from build123d import *

# Parameters (mm, degrees)
SKETCH1_R           = 3.425
HUB_DEPTH           = 2.4
SKETCH2_R           = 0.4
BOSS_EXTRUDE2_DEPTH = 1.8
SKETCH3_R           = 2.15
CUT_EXTRUDE1_DEPTH  = 0.8
SKETCH4_R           = 1.2
CUT_EXTRUDE2_DEPTH  = 17.520612
CUT_EXTRUDE3_START  = -3
CUT_EXTRUDE3_DEPTH  = 3
CIRPATTERN1_COUNT   = 20
CUT_EXTRUDE4_START  = -3
SKETCH6_R           = 2.15
CUT_EXTRUDE4_DEPTH  = 3


with BuildPart() as part:
    # Sketch1 → HUB (new body)
    with BuildSketch(Plane(origin=(0, 0, 0), x_dir=(1, 0, 0), z_dir=(0, 1, 0))):
        with Locations(Location((0, 0, 0), (0, 0, 270))):
            Circle(SKETCH1_R)
    extrude(amount=HUB_DEPTH)

    # Sketch2 → Boss-Extrude2 (add)
    with BuildSketch(Plane(origin=(0, 2.4, 0), x_dir=(1, 0, 0), z_dir=(0, 1, 0))):
        with BuildLine():
            Line((-2.875, 1.861451), (-1.85, 14))
            add(Edge.make_bspline(
                [(-1.85, 14), (-1.761904, 15.043277), (-0.882336, 15.809649), (0.882387, 15.802355), (1.755744, 15.11622), (1.85, 14)],
                knots=[0, 0, 0, 0, 0.45, 0.55, 1, 1, 1, 1], degree=3))
            Line((1.85, 14), (2.875, 1.861451))
            ThreePointArc((2.875, 1.861451), (0, -3.425), (-2.875, 1.861451))
        make_face()
        with Locations(Location((0, 14.8, 0), (0, 0, 270))):
            Circle(SKETCH2_R, mode=Mode.SUBTRACT)
        with Locations(Location((0, 12.8, 0), (0, 0, 270))):
            Circle(SKETCH2_R, mode=Mode.SUBTRACT)
        with Locations(Location((0, 10.8, 0), (0, 0, 270))):
            Circle(SKETCH2_R, mode=Mode.SUBTRACT)
        with Locations(Location((0, 8.8, 0), (0, 0, 270))):
            Circle(SKETCH2_R, mode=Mode.SUBTRACT)
        with Locations(Location((0, 6.8, 0), (0, 0, 270))):
            Circle(SKETCH2_R, mode=Mode.SUBTRACT)
        with Locations(Location((0, 4.8, 0), (0, 0, 270))):
            Circle(SKETCH2_R, mode=Mode.SUBTRACT)
    extrude(amount=BOSS_EXTRUDE2_DEPTH)

    # Sketch3 → Cut-Extrude1 (cut)
    with BuildSketch(Plane(origin=(0, 4.2, 0), x_dir=(1, 0, 0), z_dir=(0, 1, 0))):
        with Locations(Location((0, 0, 0), (0, 0, 270))):
            Circle(SKETCH3_R)
    extrude(amount=-CUT_EXTRUDE1_DEPTH, mode=Mode.SUBTRACT)

    # Sketch4 → Cut-Extrude2 (cut, through all)
    with BuildSketch(Plane(origin=(0, 3.4, 0), x_dir=(1, 0, 0), z_dir=(0, 1, 0))):
        with Locations(Location((0, 0, 0), (0, 0, 270))):
            Circle(SKETCH4_R)
    extrude(amount=-CUT_EXTRUDE2_DEPTH, mode=Mode.SUBTRACT)

    # Sketch5 → Cut-Extrude3 (cut)
    with BuildSketch(Plane.XZ.offset(CUT_EXTRUDE3_START)):
        with BuildLine():
            Line((0, 2.35), (-0.210311, 2.139689))
            ThreePointArc((-0.210311, 2.139689), (0, 2.15), (0.210311, 2.139689))
            Line((0.210311, 2.139689), (0, 2.35))
        make_face()
    cut_extrude3 = extrude(amount=CUT_EXTRUDE3_DEPTH, mode=Mode.SUBTRACT)

    # CirPattern1: Cut-Extrude3 ×20 about axis
    cirpattern1_axis = Axis((0, 0, 0), (0, 1, 0))
    for i in range(1, CIRPATTERN1_COUNT):
        add(cut_extrude3.rotate(cirpattern1_axis, i * 360 / CIRPATTERN1_COUNT), mode=Mode.SUBTRACT)

    # Sketch6 → Cut-Extrude4 (cut)
    with BuildSketch(Plane.XZ.offset(CUT_EXTRUDE4_START)):
        with Locations(Location((0, 0, 0), (0, 0, 90))):
            Circle(SKETCH6_R)
    extrude(amount=CUT_EXTRUDE4_DEPTH, mode=Mode.SUBTRACT)


solid = part.part
Work out the finished part from the listing and answer in its coordinate system (mm). A direction names the side the tool comes from. Give positions to 0.01 mm unless a question says otherwise; leave off trailing zeros. Write each loop counter-clockwise with the first axis right and the second up, starting at its lowest first coordinate (ties: lowest second). Pieces come first, ordered by that corner, then holes. Notation, with made-up numbers: M 23.25,63 L 81.25,63 A19 cw 81.25,84 Z; hole C 29,-23 d6. An arc over 180 degrees is marked long. Answer as CSV lines item,"result".
Q1. A tool of negligible diameter and unlimited length cuts with its end or side. For faces 1 (the flat face through (-1, 3, -1)), 2 (the cylindrical face through (0, 3.3, -15.2)), 3 (the cylindrical face through (-1.308, 3.806, -1.706)), from which of +Z, -Z, +X, -X, +Y, -Y can it reach the whole face along a straight path? Write none if from no direction.
A:
face 1,"-Y"
face 2,"+Y, -Y"
face 3,"+Y"
Q2. Find the intervals of material crossed by probe 1 along X at (y, z) = (3.1, 0) (3 decimals); probe 2 along X at (y, z) = (3.7, 0) (3 decimals); probe 3 along Y at (x, z) = (2, -5), in increasing order. Write a range as [from, to].
A:
probe 1,"x = [-3.425, -1.2], [1.2, 3.425]"
probe 2,"x = [-3.425, -2.15], [2.15, 3.425]"
probe 3,"y = [2.4, 4.2]"
Q3. The mould has two halves that part along X. Classify faces 4 (the flat face through (-2.37, 3.29, -7.85)), 5 (the flat face through (-1, 2.4, -9)), 6 (the cylindrical face through (0.12, 3.29, -12.42)): +X half, -X half, draft (parallel to the pull), parting line (faces both ways), or undercut.
A:
face 4,"-X half"
face 5,"draft"
face 6,"undercut"
Q4. A cutting plane is placed at B-B on z = -4.8. Write down the section's boundary in (x, y).
A:
outline,"M -2.63,2.4 L -0.4,2.4 L -0.4,4.2 L -2.63,4.2 Z; M 0.4,2.4 L 2.63,2.4 L 2.63,4.2 L 0.4,4.2 Z"
Q5. Given P1, Ø1.4, axis at x = 0, z = 0, coming from the +Y side; P2, Ø1.4, axis at x = 0.5, z = 0.5, coming from the -Y side, each flat-ended and moving along its own axis, determine where each tip first touches the part or whether it passes through.
A:
P1,"passes through"
P2,"stops at y = 3"
Q6. A cutting plane is placed at A-A on z = -8.75. Write down the section's boundary in (x, y).
A:
outline,"M -2.29,2.4 L -0.4,2.4 L -0.4,4.2 L -2.29,4.2 Z; M 0.4,2.4 L 2.29,2.4 L 2.29,4.2 L 0.4,4.2 Z"
